Can you work these out from the model? Positions are in its coordinate system, mm. Face numbers are marked on the shaded views. A direction names the side the tool comes from. Give positions to 0.01 mm unless a question says otherwise; leave off trailing zeros. Loops run counter-clockwise (first coordinate to the right, second up) from the corner with the lowest first, then second, coordinate; pieces in that order, holes last.
from build123d import *

# Parameters (mm, degrees)
EXTRUDE_1_DEPTH     = 10
SKETCH_2_R          = 2.45
EXTRUDE_2_DEPTH     = 10
SKETCH_3_R          = 1.75
CUT_EXTRUDE_1_DEPTH = 11
EXTRUDE_3_DEPTH     = 2.5
EXTRUDE_4_DEPTH     = 2.5
EXTRUDE_5_REACH     = 9.5
SKETCH_6_R          = 2.5
FILLET_1_R          = 2
SKETCH_7_W          = 6
SKETCH_7_H          = 22
EXTRUDE_6_DEPTH     = 10
FILLET_2_R          = 1
CHAMFER_1_SIZE      = 1
CHAMFER_2_SIZE      = 1
SKETCH_8_R          = 1.75
CUT_EXTRUDE_2_DEPTH = 11


with BuildPart() as part:
    # ｽｹｯﾁ1 → ﾎﾞｽ - 押し出し1 (new body)
    with BuildSketch(Plane.XY):
        with BuildLine():
            Line((-15, -25.980762114), (15, -25.980762114))
            ThreePointArc((15, -25.980762114), (0, 30), (-15, -25.980762114))
        make_face()
        with BuildLine():
            Line((-13.594396682, -20.980762114), (13.594396682, -20.980762114))
            ThreePointArc((13.594396682, -20.980762114), (0, 25), (-13.594396682, -20.980762114))
        make_face(mode=Mode.SUBTRACT)
    extrude(amount=EXTRUDE_1_DEPTH)

    # ｽｹｯﾁ2 → ﾎﾞｽ - 押し出し2 (add)
    with BuildSketch(Plane.XY):
        with BuildLine():
            Line((-13.594396682, -20.980762114), (13.594396682, -20.980762114))
            ThreePointArc((13.594396682, -20.980762114), (15.495156387, -19.618871745), (17.260361171, -18.085351317))
            Line((17.260361171, -18.085351317), (7.250462296, 3.380946094))
            ThreePointArc((7.250462296, 3.380946094), (0, 8), (-7.250462296, 3.380946094))
            Line((-7.250462296, 3.380946094), (-17.260361171, -18.085351317))
            ThreePointArc((-17.260361171, -18.085351317), (-15.495156387, -19.618871745), (-13.594396682, -20.980762114))
        make_face()
        Circle(SKETCH_2_R, mode=Mode.SUBTRACT)
    extrude(amount=EXTRUDE_2_DEPTH)

    # ｽｹｯﾁ3 → ｶｯﾄ - 押し出し1 (cut, through all)
    with BuildSketch(Plane.XY.offset(10)):
        with Locations((0, -20.980762114)):
            Circle(SKETCH_3_R)
        with Locations((-10, -20.980762114)):
            Circle(SKETCH_3_R)
    extrude(amount=-CUT_EXTRUDE_1_DEPTH, mode=Mode.SUBTRACT)

    # ｽｹｯﾁ4 → ﾎﾞｽ - 押し出し3 (add)
    with BuildSketch(Plane.XY):
        with BuildLine():
            Line((-23.452078799, -25.980762114), (-15, -25.980762114))
            ThreePointArc((-15, -25.980762114), (0, 30), (15, -25.980762114))
            Line((15, -25.980762114), (23.452078799, -25.980762114))
            ThreePointArc((23.452078799, -25.980762114), (0, 35), (-23.452078799, -25.980762114))
        make_face()
    extrude_3 = extrude(amount=EXTRUDE_3_DEPTH)

    # ｽｹｯﾁ5 → ﾎﾞｽ - 押し出し4 (add)
    with BuildSketch(Plane.XY):
        with BuildLine():
            Line((-30.333333333, 17.461067805), (-39.666666667, 1.247219129))
            ThreePointArc((-39.666666667, 1.247219129), (-40, 0), (-39.666666667, -1.247219129))
            Line((-39.666666667, -1.247219129), (-30.333333333, -17.461067805))
            Line((-30.333333333, -17.461067805), (-30.333333333, 17.461067805))
        make_face()
    extrude_4 = extrude(amount=EXTRUDE_4_DEPTH)

    # ﾐﾗｰ2: ﾎﾞｽ - 押し出し3, ﾎﾞｽ - 押し出し4 across plane
    add(extrude_3.mirror(Plane(origin=(0, 0, 5), x_dir=(1, 0, 0), z_dir=(0, 0, -1))))
    add(extrude_4.mirror(Plane(origin=(0, 0, 5), x_dir=(1, 0, 0), z_dir=(0, 0, -1))))

    # ｽｹｯﾁ6 → ﾎﾞｽ - 押し出し5 (add, up to next)
    with BuildSketch(Plane.XY.offset(2.5), mode=Mode.PRIVATE) as extrude_5_sk1:
        with Locations((-37.5, 0)):
            Circle(SKETCH_6_R)
    extrude_5_tool1 = extrude(extrude_5_sk1.sketch, amount=EXTRUDE_5_REACH, mode=Mode.PRIVATE) - part.part
    add(extrude_5_tool1.solids().sort_by_distance((-37.5, 0, 2.5))[0])

    # ﾌｨﾚｯﾄ1
    fillet_1_edges = [part.edges().sort_by_distance(p)[0] for p in [
        (-17.260361171, -18.085351317, 5),
        (17.260361171, -18.085351317, 5),
    ]]
    fillet(fillet_1_edges, radius=FILLET_1_R)

    # ｽｹｯﾁ7 → ﾎﾞｽ - 押し出し6 (add)
    with BuildSketch(Plane.XY.offset(10)):
        with Locations((0, 16)):
            Rectangle(SKETCH_7_W, SKETCH_7_H)
    extrude(amount=-EXTRUDE_6_DEPTH)

    # ﾌｨﾚｯﾄ2
    fillet_2_edges = [part.edges().sort_by_distance(p)[0] for p in [
        (3, 7.416198487, 5),
        (-3, 7.416198487, 5),
        (-3, 24.819347292, 5),
        (3, 24.819347292, 5),
    ]]
    fillet(fillet_2_edges, radius=FILLET_2_R)

    # 面取り1
    chamfer_1_edges = [part.edges().sort_by_distance(p)[0] for p in [
        (11.627163615, -6.004920172, 0),
        (11.627163615, -6.004920172, 10),
        (23.403223211, 8.791424421, 0),
        (23.403223211, 8.791424421, 10),
        (17.568783294, -16.530152165, 0),
        (17.568783294, -16.530152165, 10),
        (-17.568783294, -16.530152165, 0),
        (-17.568783294, -16.530152165, 10),
        (-3, 15.86328844, 10),
        (-3, 15.86328844, 0),
        (-23.403223211, 8.791424421, 10),
        (-23.403223211, 8.791424421, 0),
        (3, 15.86328844, 0),
        (3, 15.86328844, 10),
        (-5.724946981, 5.587931824, 10),
        (-5.724946981, 5.587931824, 0),
        (-3.354502776, 24.428081748, 0),
        (-3.354502776, 24.428081748, 10),
        (3.354502776, 24.428081748, 10),
        (3.354502776, 24.428081748, 0),
        (3.150163414, 7.535211472, 10),
        (3.150163414, 7.535211472, 0),
        (-3.150163414, 7.535211472, 0),
        (-3.150163414, 7.535211472, 10),
        (5.724946981, 5.587931824, 10),
        (-11.627163615, -6.004920172, 10),
        (5.724946981, 5.587931824, 0),
        (-11.627163615, -6.004920172, 0),
    ]]
    chamfer(chamfer_1_edges, length=CHAMFER_1_SIZE)

    # 面取り2
    chamfer_2_edges = [part.edges().sort_by_distance(p)[0] for p in [
        (21.991727141, 27.227999143, 0),
        (-27.227999143, -21.991727141, 0),
        (-35, 9.354143467, 0),
        (-40, 0, 0),
        (-35, -9.354143467, 0),
        (21.991727141, 27.227999143, 10),
        (-27.227999143, -21.991727141, 10),
        (-35, 9.354143467, 10),
        (-40, 0, 10),
        (-35, -9.354143467, 10),
    ]]
    chamfer(chamfer_2_edges, length=CHAMFER_2_SIZE)

    # ｽｹｯﾁ8 → ｶｯﾄ - 押し出し2 (cut, through all)
    with BuildSketch(Plane.XY.offset(10)):
        with Locations((-5, -12.980762114)):
            Circle(SKETCH_8_R)
    extrude(amount=-CUT_EXTRUDE_2_DEPTH, mode=Mode.SUBTRACT)


solid = part.part
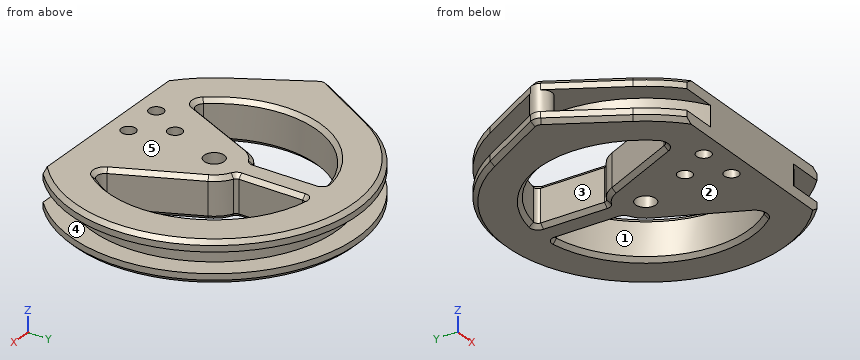
(1) Suppose I cut it at B-B on z = 4.75. List the corners of the cut face in (x, y) for me.
Returned:
outline: circle Ø5 at (-37.5, 0); (-15, -25.98) - (15, -25.98) arc R30 ccw (long way) to start; hole (-19.37, -15.81) arc R2 ccw to (-16, -15.39) - (-7.25, 3.38) arc R8 cw to (-3.56, 7.17) arc R1 ccw to (-3, 8.06) - (-3, 23.66) arc R1 ccw to (-4.17, 24.65) arc R25 ccw to start; hole circle Ø3.5 at (-10, -20.98); hole circle Ø3.5 at (-5, -12.98); hole circle Ø4.9 at (0, 0); hole circle Ø3.5 at (0, -20.98); hole (3, 8.06) arc R1 ccw to (3.56, 7.17) arc R8 cw to (7.25, 3.38) - (16, -15.39) arc R2 ccw to (19.37, -15.81) arc R25 ccw to (4.17, 24.65) arc R1 ccw to (3, 23.66) - close
(2) Suppose I cut it at A-A on x = 0. List the corners of the cut face in (y, z) for me.
Returned:
outline: (-25.98, 0) - (-22.73, 0) - (-22.73, 10) - (-25.98, 10) - close; (-19.23, 0) - (-2.45, 0) - (-2.45, 10) - (-19.23, 10) - close; (2.45, 0) - (34, 0) - (35, 1) - (35, 2.5) - (30, 2.5) - (30, 7.5) - (35, 7.5) - (35, 9) - (34, 10) - (2.45, 10) - close
(3) Suppose I cut it at C-C on x = -37.5. List the corners of the cut face in (y, z) for me.
Returned:
outline: (-5.01, 1) - (-3.01, 0) - (3.01, 0) - (5.01, 1) - (5.01, 2.5) - (2.5, 2.5) - (2.5, 7.5) - (5.01, 7.5) - (5.01, 9) - (3.01, 10) - (-3.01, 10) - (-5.01, 9) - (-5.01, 7.5) - (-2.5, 7.5) - (-2.5, 2.5) - (-5.01, 2.5) - close
(4) Will these pins go through, and if not, where does the flat tip stop? P1, Ø2.5, axis at y = 15.5, z = 6.5, coming from the -X side; P2, Ø6, axis at y = 5.5, z = 7, coming from the +X side; P3, Ø4, axis at y = 18, z = 6.5, coming from the +X side; P4, Ø3, axis at x = 0, y = -20.98, coming from the -Z side.
Returned:
P1: stops at x = -31.89
P2: stops at x = 34.91
P3: stops at x = 30.99
P4: passes through
(5) Which directions (+Z, -Z, +X, -X, +Y, -Y) give clear straight access to the entire face, cutting with the end or side of a thin tool? Please do the marked faces 3, 4 and 5.
Returned:
face 3: +Z, -Z
face 4: none
face 5: +Z, +X, -X, +Y, -Y
(6) Thinking about a two-plate mould opening in X: for the marked faces 1 and 2, which applies, pulls with the +X half, pulls with the -X half, needs draft (parallel to the pull), parting line crosses it, or undercut?
Returned:
face 1: undercut
face 2: needs draft
(7) Suppose I cut it at D-D on y = 19. Give the number of separate pieces and of enclosed holes in the cut face, plus the area to 3 significant figures.
Returned:
separate pieces: 3
enclosed holes: 0
area: 254 mm2
(8) Please list where these lines run through material, in increasing order: probe 1 along Z at (x, y) = (-33, 7); probe 2 along Y at (x, z) = (-1.5, 3.25); probe 3 along X at (y, z) = (18, 6.75).
Returned:
probe 1: z = 0 to 2.5, 7.5 to 10
probe 2: y = -25.98 to -21.88, -20.08 to -1.94, 1.94 to 29.96
probe 3: x = -24 to -17.35, -3 to 3, 17.35 to 24
